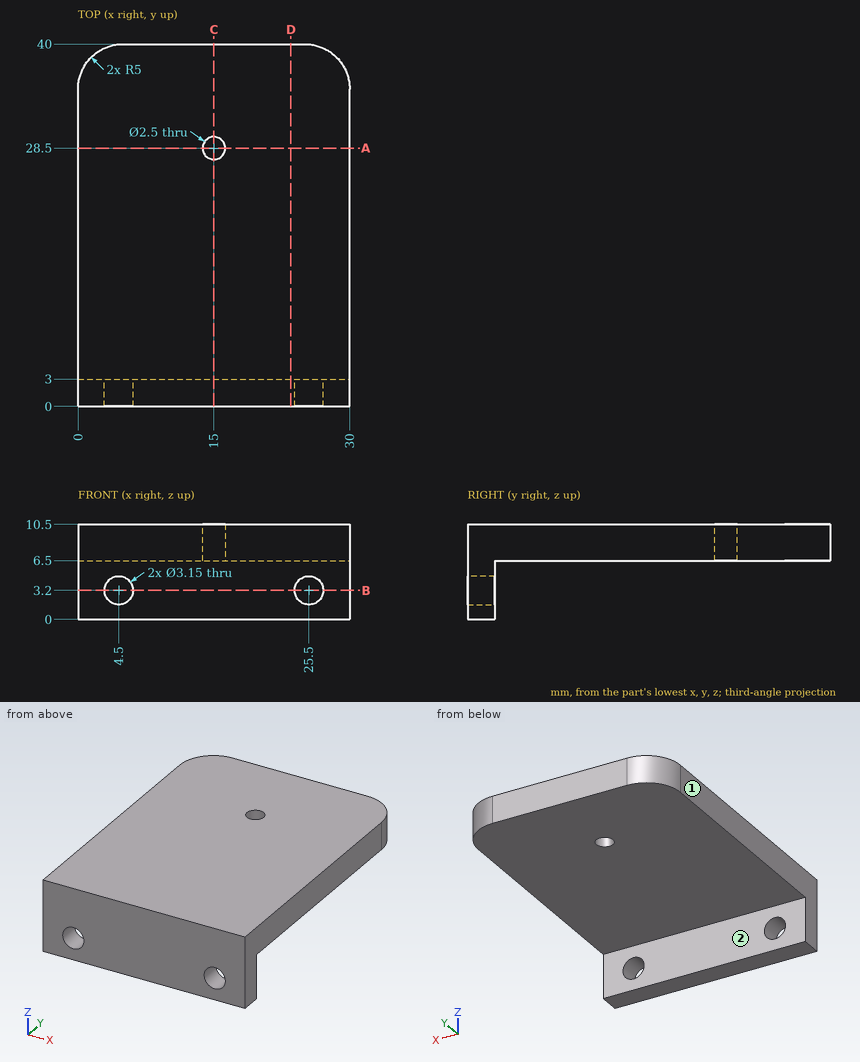
Part print with two shaded views. Sizes in mm from the minimum x, y, z corner. A direction names the side the tool comes from. Give positions to 0.01 mm unless a question says otherwise; leave off trailing zeros. Write each loop counter-clockwise with the first axis right and the second up, starting at its lowest first coordinate (ties: lowest second). Pieces come first, ordered by that corner, then holes.
1) Cut at A-A on y = 28.5. Write the cut outline in (x, z).
Resolved:
outline: (0, 6.5) - (13.75, 6.5) - (13.75, 10.5) - (0, 10.5) - close; (16.25, 6.5) - (30, 6.5) - (30, 10.5) - (16.25, 10.5) - close
2) Cut at C-C on x = 15. Write the cut outline in (y, z).
Resolved:
outline: (0, 0) - (3, 0) - (3, 6.5) - (27.25, 6.5) - (27.25, 10.5) - (0, 10.5) - close; (29.75, 6.5) - (40, 6.5) - (40, 10.5) - (29.75, 10.5) - close
3) Cut at D-D on x = 23.5. Write the cut outline in (y, z), then the cut area to 4 significant figures.
Resolved:
outline: (0, 0) - (3, 0) - (3, 6.5) - (40, 6.5) - (40, 10.5) - (0, 10.5) - close
area: 179.5 mm2
4) Which spindle directions (+Z, -Z, +X, -X, +Y, -Y) get a long thin tool onto all of the face, cutting with end or side? Do the marked faces 1 and 2. Say none if no direction does.
Resolved:
face 1: +Z, -Z, -X, +Y, -Y
face 2: -Z, +X, -X, +Y
5) Cut at B-B on z = 3.2. Write the cut outline in (x, y) (3 decimals), then the cut area to 3 significant figures.
Resolved:
outline: (0, 0) - (2.925, 0) - (2.925, 3) - (0, 3) - close; (6.075, 0) - (23.925, 0) - (23.925, 3) - (6.075, 3) - close; (27.075, 0) - (30, 0) - (30, 3) - (27.075, 3) - close
area: 71.1 mm2
6) Pin check, flat tips, straight feed: pin 1 (3 mm diameter, centred on x = 10, z = 3.5, fed in from +Y); pin 2 (2 mm diameter, centred on y = 4.5, z = 8, fed in from -X); pin 3 (10 mm diameter, centred on x = 9.5, y = 16.5, fed in from -Z); pin 4 (2 mm diameter, centred on x = 15, y = 28.5, fed in from +Z). Stop position of each tip, or through.
Resolved:
pin 1: stops at y = 3
pin 2: stops at x = 0
pin 3: stops at z = 6.5
pin 4: passes through
7) Probe L1, parallel to X at y = 0.75, z = 3.2 (3 decimals); L2, parallel to Y at x = 15, z = 7.9; L3, parallel to Y at x = 20, z = 1.75. List the from-to ranges inside material, lowest first.
Resolved:
L1: x = 0 to 2.925, 6.075 to 23.925, 27.075 to 30
L2: y = 0 to 27.25, 29.75 to 40
L3: y = 0 to 3
